The model under review builds one solid part; all positions refer to its coordinate system, in mm. A direction names the side the tool comes from. Round coordinates to 2 decimals unless told otherwise and drop trailing zeros. Write each loop counter-clockwise with the first axis right and the second up, starting at its lowest first coordinate (ties: lowest second). Pieces come first, ordered by that corner, then holes. Notation, with made-up numbers: (3.25, 16.5) -> (27.25, 16.5) arc R18 ccw to (27.25, 46.5) -> close; hole circle Ø6 at (-18, 29.25). An arc over 180 degrees is marked (long way). Return JSON: item names as keys, results as strings. Group by question number.
1. Take a section at B-B, the plane y = 34. Write out the cut boundary in (x, z).
2. Mouldability with a two-part tool opening along X and no side actions: class faces 6 (the flat face through (16, 35, 10)), 7 (the flat face through (-20, -1.7, 1.6)), 8 (the flat face through (20, -2.8, 1.6)), 9 (the flat face through (-18, -36, 14)) as pulls with the +X half, pulls with the -X half, needs draft (parallel to the pull), parting line crosses it, or undercut.
3. Clearance check with flat-ended pins moving along their axes: P1, Ø6, axis at x = -11, z = 11.5, coming from the -Y side; P2, Ø5.5, axis at x = -18.5, z = 6.5, coming from the -Y side; P3, Ø2.5, axis at x = -7.5, y = -39.5, coming from the +Z side. State where each tip first meets the part, or that it passes through.
4. Take a section at A-A, the plane x = -6.5. Write out the cut boundary in (y, z), then the cut area to 3 significant figures.
5. For line 1 along X through (y, z) = (-35, 3.25); line 2 along Y through (x, z) = (-16, 3.5); line 3 along Y through (x, z) = (18, 13.75), list the stretches that pass through material, from the lowest coordinate up. Write a range as from..to.
6. Tool access review of faces 1 (the flat face through (0, -2, 0)), 2 (the cylindrical face through (-18.7, -36.9, 12)), 3 (the flat face through (17, 31.5, 6)), 4 (the flat face through (-18, -38.5, 6)), 5 (the flat face through (0, 2.5, 1)): name each direction out of +Z, -Z, +X, -X, +Y, -Y from which nothing blocks a thin tool from reaching the whole face with its end or side.
7. Take a section at D-D, the plane x = -17.5. Write out the cut boundary in (y, z), then the cut area to 3 significant figures.
8. Take a section at C-C, the plane z = 8.25. Write out the cut boundary in (x, y).
from build123d import *

# Parameters (mm, degrees)
F0_W     = 5
F0_H     = 29
F0_H_2   = 31
F0_H_3   = 5
F0_R     = 1.5
F0_W_2   = 30
F0_H_4   = 2.5
F1_DEPTH = 2
F2_DEPTH = 10
F3_DEPTH = 14


with BuildPart() as f1:
    # F0 (on Top) → F1 (new body)
    with BuildSketch(Plane.XY):
        Polygon((-20, -41), (20, -41), (20, -38.5), (15, -38.5), (-15, -38.5), (-20, -38.5), align=None)
        with Locations((-17.5, 17)):
            Rectangle(F0_W, F0_H)
        with Locations((-17.5, -18)):
            Rectangle(F0_W, F0_H_2)
        with Locations((-17.5, 0)):
            Rectangle(F0_W, F0_H_3)
        with Locations((17.5, 17)):
            Rectangle(F0_W, F0_H)
        with Locations((17.5, -18)):
            Rectangle(F0_W, F0_H_2)
        with Locations((17.5, 0)):
            Rectangle(F0_W, F0_H_3)
        with Locations((-17.5, 34)):
            Rectangle(F0_W, F0_H_3)
        with Locations((-17.5, 34)):
            Circle(F0_R, mode=Mode.SUBTRACT)
        with Locations((17.5, 34)):
            Rectangle(F0_W, F0_H_3)
        with Locations((17.5, 34)):
            Circle(F0_R, mode=Mode.SUBTRACT)
        Polygon((15, -38.5), (20, -38.5), (20, -33.5), (15, -33.5), (15, -36), align=None)
        with Locations((17.5, -36)):
            Circle(F0_R, mode=Mode.SUBTRACT)
        Polygon((-20, -33.5), (-20, -38.5), (-15, -38.5), (-15, -36), (-15, -33.5), align=None)
        with Locations((-17.5, -36)):
            Circle(F0_R, mode=Mode.SUBTRACT)
        with Locations((-17.5, 34)):
            Circle(F0_R)
        with Locations((17.5, 34)):
            Circle(F0_R)
        Rectangle(F0_W_2, F0_H_3)
        with Locations((-17.5, -36)):
            Circle(F0_R)
        with Locations((17.5, -36)):
            Circle(F0_R)
        with Locations((0, -37.25)):
            Rectangle(F0_W_2, F0_H_4)
    extrude(amount=F1_DEPTH)

    # F0 (on Top) → F2 (join)
    with BuildSketch(Plane.XY):
        with Locations((17.5, 34)):
            Rectangle(F0_W, F0_H_3)
        with Locations((17.5, 34)):
            Circle(F0_R, mode=Mode.SUBTRACT)
        with Locations((17.5, 34)):
            Circle(F0_R)
        with Locations((-17.5, 34)):
            Rectangle(F0_W, F0_H_3)
        with Locations((-17.5, 34)):
            Circle(F0_R, mode=Mode.SUBTRACT)
        with Locations((-17.5, 34)):
            Circle(F0_R)
        Polygon((15, -38.5), (20, -38.5), (20, -33.5), (15, -33.5), (15, -36), align=None)
        with Locations((17.5, -36)):
            Circle(F0_R, mode=Mode.SUBTRACT)
        with Locations((17.5, -36)):
            Circle(F0_R)
        Polygon((-20, -33.5), (-20, -38.5), (-15, -38.5), (-15, -36), (-15, -33.5), align=None)
        with Locations((-17.5, -36)):
            Circle(F0_R, mode=Mode.SUBTRACT)
        with Locations((-17.5, -36)):
            Circle(F0_R)
    extrude(amount=F2_DEPTH)

    # F0 (on Top) → F3 (join)
    with BuildSketch(Plane.XY):
        with Locations((17.5, 34)):
            Circle(F0_R)
        with Locations((-17.5, 34)):
            Circle(F0_R)
        with Locations((17.5, -36)):
            Circle(F0_R)
        with Locations((-17.5, -36)):
            Circle(F0_R)
    extrude(amount=F3_DEPTH)


solid = f1.part
Output:
{
 "1": {"outline": "(-20, 0) -> (-15, 0) -> (-15, 10) -> (-16, 10) -> (-16, 14) -> (-19, 14) -> (-19, 10) -> (-20, 10) -> close; (15, 0) -> (20, 0) -> (20, 10) -> (19, 10) -> (19, 14) -> (16, 14) -> (16, 10) -> (15, 10) -> close"},
 "2": {"face 6": "undercut", "face 7": "pulls with the -X half", "face 8": "pulls with the +X half", "face 9": "needs draft"},
 "3": {"P1": "passes through", "P2": "stops at y = -38.5", "P3": "stops at z = 2"},
 "4": {"outline": "(-41, 0) -> (-36, 0) -> (-36, 2) -> (-41, 2) -> close; (-2.5, 0) -> (2.5, 0) -> (2.5, 2) -> (-2.5, 2) -> close", "area": "20.0 mm^2"},
 "5": {"line 1": "x = -20..-15, 15..20", "line 2": "y = -38.5..-33.5, 31.5..36.5", "line 3": "y = -37.41..-34.59, 32.59..35.41"},
 "6": {"face 1": "-Z, +X, -X, +Y, -Y", "face 2": "+Z", "face 3": "+Z, +X, -X", "face 4": "+Z, +X, -X, -Y", "face 5": "+Z, -Z, +Y"},
 "7": {"outline": "(-41, 0) -> (36.5, 0) -> (36.5, 10) -> (35.5, 10) -> (35.5, 14) -> (32.5, 14) -> (32.5, 10) -> (31.5, 10) -> (31.5, 2) -> (-33.5, 2) -> (-33.5, 10) -> (-34.5, 10) -> (-34.5, 14) -> (-37.5, 14) -> (-37.5, 10) -> (-38.5, 10) -> (-38.5, 2) -> (-41, 2) -> close", "area": "259 mm^2"},
 "8": {"outline": "(-20, -38.5) -> (-15, -38.5) -> (-15, -33.5) -> (-20, -33.5) -> close; (-20, 31.5) -> (-15, 31.5) -> (-15, 36.5) -> (-20, 36.5) -> close; (15, -38.5) -> (20, -38.5) -> (20, -33.5) -> (15, -33.5) -> close; (15, 31.5) -> (20, 31.5) -> (20, 36.5) -> (15, 36.5) -> close"}
}
